```python
from build123d import *

# Parameters (mm, degrees)
BOSS_EXTRUDE1_DEPTH = 60
SKETCH2_R           = 2.5
CUT_EXTRUDE1_DEPTH  = 10
SKETCH3_R           = 2.5
CUT_EXTRUDE2_DEPTH  = 10


with BuildPart() as part:
    # Sketch1 → Boss-Extrude1 (new body)
    with BuildSketch(Plane.XY):
        Polygon((0, 0), (0, 20), (2, 20), (2, 2), (30, 2), (30, 0), align=None)
    extrude(amount=BOSS_EXTRUDE1_DEPTH)

    # Sketch2 → Cut-Extrude1 (cut)
    with BuildSketch(Plane(origin=(0, 2, 0), x_dir=(1, 0, 0), z_dir=(0, 1, 0))):
        with Locations((20, -30)):
            Circle(SKETCH2_R)
        with Locations((20, -10)):
            Circle(SKETCH2_R)
        with Locations((20, -50)):
            Circle(SKETCH2_R)
    extrude(amount=-CUT_EXTRUDE1_DEPTH, mode=Mode.SUBTRACT)

    # Sketch3 → Cut-Extrude2 (cut)
    with BuildSketch(Plane(origin=(2, 0, 0), x_dir=(0, 0, -1), z_dir=(1, 0, 0))):
        with Locations((-30, 7)):
            Circle(SKETCH3_R)
        with Locations((-10, 7)):
            Circle(SKETCH3_R)
        with Locations((-50, 7)):
            Circle(SKETCH3_R)
    extrude(amount=-CUT_EXTRUDE2_DEPTH, mode=Mode.SUBTRACT)


solid = part.part
```
Can you work these out from the model? Positions are in its coordinate system, mm. A direction names the side the tool comes from. Coordinates: 2 decimals unless noted, no trailing zeros. Loops run counter-clockwise (first coordinate to the right, second up) from the corner with the lowest first, then second, coordinate; pieces in that order, holes last. Notation, with made-up numbers: (19.5, 74.5) - (78.5, 74.5) arc R32 ccw to (78.5, 106.5) - close; hole circle Ø2 at (-23.75, -8.5). An arc over 180 degrees is marked (long way). Answer as CSV lines item,"result". Start each with the question number.
1) Suppose I cut it at A-A (x = 20). Please give me the cut outline in (y, z), plus the area to 3 significant figures.
2) Thinking about a two-plate mould opening in Y: for faces 1 (the flat face through (8, 1, 60)), 2 (the flat face through (16, 2, 30)), 3 (the cylindrical face through (1, 7.1, 32.5)), which applies, pulls with the +Y half, pulls with the -Y half, needs draft (parallel to the pull), parting line crosses it, or undercut?
3) For pin 1 (8 mm diameter, centred on x = 20, z = 30, fed in from +Y); pin 2 (8 mm diameter, centred on y = 7, z = 10, fed in from +X); pin 3 (4 mm diameter, centred on y = 7, z = 50, fed in from -X), each with a flat end and sliding along its axis, tell me the tip position at first contact or that it passes through.
4) Suppose I cut it at D-D (z = 35.5). Please give me the cut outline in (x, y), plus the area to 3 significant figures.
5) I need wall thicknesses on line 1 (Z direction, x = 20, y = 1.3); line 2 (Y direction, x = 1.25, z = 30); line 3 (X direction, y = 1.25, z = 30). Which ranges of each line are inside material? Lowest first, please. Write a range as from..to.
6) Which directions (+Z, -Z, +X, -X, +Y, -Y) give clear straight access to the entire face, cutting with the end or side of a thin tool? Please do faces 4 (the flat face through (2, 11, 30)), 5 (the cylindrical face through (18, 1, 11.5)).
7) Suppose I cut it at C-C (z = 10). Please give me the cut outline in (x, y), plus the area to 3 significant figures.
Check result:
1,outline,"(0, 0) - (2, 0) - (2, 7.5) - (0, 7.5) - close; (0, 12.5) - (2, 12.5) - (2, 27.5) - (0, 27.5) - close; (0, 32.5) - (2, 32.5) - (2, 47.5) - (0, 47.5) - close; (0, 52.5) - (2, 52.5) - (2, 60) - (0, 60) - close"
1,area,"90.0 mm²"
2,face 1,"needs draft"
2,face 2,"pulls with the +Y half"
2,face 3,"undercut"
3,pin 1,"stops at y = 2"
3,pin 2,"stops at x = 2"
3,pin 3,"passes through"
4,outline,"(0, 0) - (30, 0) - (30, 2) - (2, 2) - (2, 20) - (0, 20) - close"
4,area,"96.0 mm²"
5,line 1,"z = 0..7.5, 12.5..27.5, 32.5..47.5, 52.5..60"
5,line 2,"y = 0..4.5, 9.5..20"
5,line 3,"x = 0..17.5, 22.5..30"
6,face 4,"+Z, -Z, +X, +Y"
6,face 5,"+Y, -Y"
7,outline,"(0, 0) - (17.5, 0) - (17.5, 2) - (2, 2) - (2, 4.5) - (0, 4.5) - close; (0, 9.5) - (2, 9.5) - (2, 20) - (0, 20) - close; (22.5, 0) - (30, 0) - (30, 2) - (22.5, 2) - close"
7,area,"76.0 mm²"
